from build123d import *

# Parameters (mm, degrees)
F1_DEPTH = 762


# Not quite as in the source:
# - a feature names something its author has since deleted; it is built from what else it names


with BuildPart() as f1:
    # F0 (on Right) → F1 (new body)
    with BuildSketch(Plane.YZ):
        with BuildLine():
            ThreePointArc((-76.2, 6.35), (-102.0787858137, -3.6681324257), (-127, -15.875))
            ThreePointArc((-127, -15.875), (-101.6930614476, -18.9514831615), (-76.2, -19.05))
            Line((-76.2, -19.05), (-76.2, -17.4625))
            Line((-76.2, -17.4625), (-76.2, 6.35))
        make_face()
        with BuildLine():
            Line((127, -19.05), (-25.4, 19.05))
            ThreePointArc((-25.4, 19.05), (-51.0583154566, 13.7332618264), (-76.2, 6.35))
            Line((-76.2, 6.35), (-76.2, -17.4625))
            Line((-76.2, -17.4625), (-76.2, -19.05))
            Line((-76.2, -19.05), (127, -19.05))
        make_face()
    extrude(amount=F1_DEPTH)


solid = f1.part
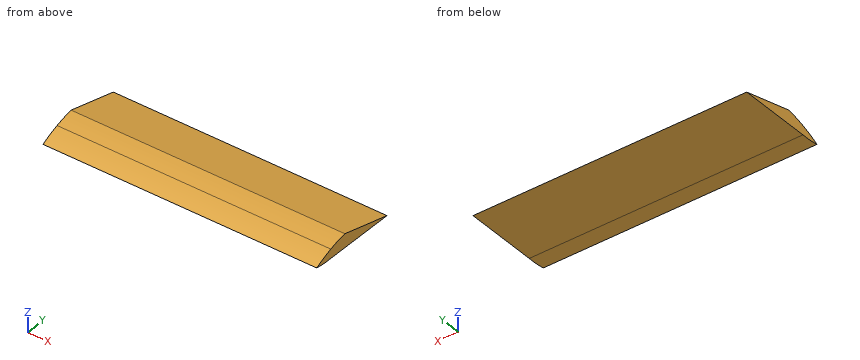
Source: CAD feature listing. Evaluate the final solid. Frame: model axes, mm. Coordinates: 2 decimals unless noted, no trailing zeros. Loops run counter-clockwise (first coordinate to the right, second up) from the corner with the lowest first, then second, coordinate; pieces in that order, holes last. Notation, with made-up numbers: (-0.75, 44) - (29.25, 44) arc R24 ccw to (29.25, 75) - close; hole circle Ø7 at (60.5, -4). An arc over 180 degrees is marked (long way). One line per question, with ' | ' between items.
1) Line query: line 1 along Z through (x, y) = (553, -100.5); line 2 along Z through (x, y) = (377, -86.5). Output: solid intervals per line, ascending.
Report:
line 1: z = -19.02 to -2.98 | line 2: z = -19.37 to 2.67
2) First-contact query: P1, Ø1.5, axis at x = 284, y = 83, coming from the -Z side. Flat tip, straight axial feed; report the tip coordinate or a pass-through.
Report:
P1: stops at z = -19.05
3) Section C-C, the plane z = 0.5. Return loops of the section in (x, y).
Report:
outline: (0, -92.1) - (762, -92.1) - (762, 48.8) - (0, 48.8) - close
4) Section B-B, the plane y = 90. Return loops of the section in (x, z).
Report:
outline: (0, -19.05) - (762, -19.05) - (762, -9.8) - (0, -9.8) - close
